Here's how the part is built. I have some questions about the finished solid (model axes, mm). A direction names the side the tool comes from. Round coordinates to 2 decimals unless told otherwise and drop trailing zeros. Loops run counter-clockwise (first coordinate to the right, second up) from the corner with the lowest first, then second, coordinate; pieces in that order, holes last. Notation, with made-up numbers: M 89,-34 L 136,-34 A23 cw 136,-3 Z; hole C -27,37.5 d10. An arc over 180 degrees is marked long. Answer as a JSON object with one key per item and string values.
from build123d import *

# Parameters (mm, degrees)
SKETCH_1_W      = 105
SKETCH_1_H      = 102.5
EXTRUDE_1_DEPTH = 2.5
EXTRUDE_2_DEPTH = 10


with BuildPart() as part:
    # Эскиз1 → Бобышка-Вытянуть1 (new body)
    with BuildSketch(Plane(origin=(0, 0, 0), x_dir=(1, 0, 0), z_dir=(0, 1, 0))):
        with Locations((57.513799089, -63.375984423)):
            Rectangle(SKETCH_1_W, SKETCH_1_H)
    extrude(amount=EXTRUDE_1_DEPTH)

    # Эскиз2 → Бобышка-Вытянуть2 (add)
    with BuildSketch(Plane(origin=(0, 2.5, 0), x_dir=(1, 0, 0), z_dir=(0, 1, 0))):
        Polygon((5.013799089, -12.125984423), (110.013799089, -12.125984423), (110.013799089, -114.625984423), (107.763799089, -114.625984423), (107.763799089, -112.909428801), (107.763799089, -14.425984423), (7.263799089, -14.425984423), (7.263799089, -112.909428801), (7.263799089, -114.625984423), (5.013799089, -114.625984423), align=None)
    extrude(amount=EXTRUDE_2_DEPTH)


solid = part.part
Item 1: I want a section at B-B, the plane y = 6. Please give me the cut outline in (x, z).
Resolved:
{"outline": "M 5.01,12.13 L 110.01,12.13 L 110.01,114.63 L 107.76,114.63 L 107.76,14.43 L 7.26,14.43 L 7.26,114.63 L 5.01,114.63 Z"}
Item 2: Please list where these lines run through material, in increasing order: probe 1 along X at (y, z) = (4.5, 79); probe 2 along Y at (x, z) = (12, 65); probe 3 along Z at (x, y) = (46.5, 7.75). Write a range as from..to.
Resolved:
{"probe 1": "5.01..7.26, 107.76..110.01", "probe 2": "0..2.5", "probe 3": "12.13..14.43"}
Item 3: I want a section at A-A, the plane z = 88.5. Please give me the cut outline in (x, y), then the cut area to 4 significant figures.
Resolved:
{"outline": "M 5.01,0 L 110.01,0 L 110.01,12.5 L 107.76,12.5 L 107.76,2.5 L 7.26,2.5 L 7.26,12.5 L 5.01,12.5 Z", "area": "307.5 mm²"}
Item 4: I'm going to push a flat-ended pin straight in: pin 1 Ø6 at (x, z) = (16, 91.5) entering from +Y. Where does the tip first touch, or does it pass through?
Resolved:
{"pin 1": "y = 2.5"}
Item 5: If we mould it in two halves opening along X, with no side actions, what happens to faces 1 (the face through (5.014, 6, 64)), 2 (the face through (57, 6, 12.126)), 3 (the face through (7.264, 7, 65))? For each: pulls with the +X half, pulls with the -X half, needs draft (parallel to the pull), parting line crosses it, or undercut.
Resolved:
{"face 1": "pulls with the -X half", "face 2": "needs draft", "face 3": "undercut"}
Item 6: On a 3-axis mill with a long thin cutter (end or side, diameter ignored), from which of +Z, -Z, +X, -X, +Y, -Y can I reach the whole of each face in a straight line? I mean faces 4 (the face through (58, 12.5, 14)), 5 (the face through (57, 2.5, 64)). Say none if no direction works.
Resolved:
{"face 4": "+Z, -Z, +X, -X, +Y", "face 5": "+Z, +Y"}
Item 7: I want a section at C-C, the plane x = 82.5. Please give me the cut outline in (y, z).
Resolved:
{"outline": "M 0,12.13 L 12.5,12.13 L 12.5,14.43 L 2.5,14.43 L 2.5,114.63 L 0,114.63 Z"}
